Geometry: final body of the model. Coordinates: model frame, mm. Face numbers are marked on the shaded views. A direction names the side the tool comes from. Round coordinates to 2 decimals unless told otherwise and drop trailing zeros. Write each loop counter-clockwise with the first axis right and the second up, starting at its lowest first coordinate (ties: lowest second). Pieces come first, ordered by that corner, then holes. Notation, with made-up numbers: (-38, -7.5) -> (15, -7.5) arc R22 ccw to (15, 15.5) -> close; hole circle Ø8 at (72, 4.25). An arc over 180 degrees is marked (long way). One line per item, written item: value. Start each with the question number.
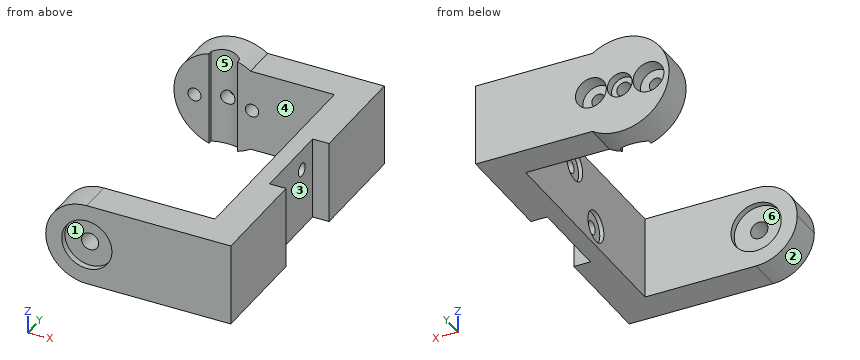
from build123d import *

# Parameters (mm, degrees)
SZKIC1_W                        = 45
SZKIC1_H                        = 20
SZKIC1_R                        = 2.1
DODANIE_WYCI_GNI_CIE1_DEPTH     = 8
SZKIC2_R                        = 6.1
WYTNIJ_WYCI_GNI_CIE1_DEPTH      = 1.5
WYTNIJ_WYCI_GNI_CIE2_START      = -1.5
SZKIC3_R                        = 6.1
WYTNIJ_WYCI_GNI_CIE2_DEPTH      = 1.5
SZKIC4_W                        = 8
SZKIC4_H                        = 20
DODANIE_WYCI_GNI_CIE2_DEPTH     = 56
ZAOKR_GLENIE1_R                 = 10
DODANIE_WYCI_GNI_CIE3_DEPTH     = 8
WYTNIJ_WYCI_GNI_CIE3_REACH      = 82.951
SZKIC6_R                        = 1.6
SZKIC7_R                        = 3.75
WYTNIJ_WYCI_GNI_CIE4_DEPTH      = 3.5
WYTNIJ_WYCI_GNI_CIE5_REACH      = 85.576
WYTNIJ_WYCI_GNI_CIE5_END_RADIUS = 12
SZKIC10_R                       = 3
WYTNIJ_WYCI_GNI_CIE6_DEPTH      = 2
WYTNIJ_WYCI_GNI_CIE7_REACH      = 81.177
WYTNIJ_WYCI_GNI_CIE7_END_RADIUS = 5
SZKIC11_R                       = 1.75
SZKIC12_W                       = 20
SZKIC12_H                       = 20.2
WYTNIJ_WYCI_GNI_CIE8_DEPTH      = 4
WYTNIJ_WYCI_GNI_CIE9_REACH      = 86.717
SZKIC13_R                       = 1.6
SZKIC14_R                       = 3.75
WYTNIJ_WYCI_GNI_CIE10_DEPTH     = 1


with BuildPart() as part:
    # Szkic1 → Dodanie-wyciągnięcie1 (new body)
    with BuildSketch(Plane(origin=(0, 0, 0), x_dir=(1, 0, 0), z_dir=(0, 1, 0))):
        with Locations((12.5, 0)):
            Rectangle(SZKIC1_W, SZKIC1_H)
        with Locations(Location((0, 0, 0), (0, 0, 270))):
            Circle(SZKIC1_R, mode=Mode.SUBTRACT)
    extrude(amount=DODANIE_WYCI_GNI_CIE1_DEPTH)

    # Szkic2 → Wytnij-wyciągnięcie1 (cut)
    with BuildSketch(Plane(origin=(0, 8, 0), x_dir=(1, 0, 0), z_dir=(0, 1, 0))):
        with Locations(Location((0, 0, 0), (0, 0, 270))):
            Circle(SZKIC2_R)
    extrude(amount=-WYTNIJ_WYCI_GNI_CIE1_DEPTH, mode=Mode.SUBTRACT)

    # Szkic3 → Wytnij-wyciągnięcie2 (cut)
    with BuildSketch(Plane.XZ.offset(WYTNIJ_WYCI_GNI_CIE2_START)):
        with Locations(Location((0, 0, 0), (0, 0, 90))):
            Circle(SZKIC3_R)
    extrude(amount=WYTNIJ_WYCI_GNI_CIE2_DEPTH, mode=Mode.SUBTRACT)

    # Szkic4 → Dodanie-wyciągnięcie2 (add)
    with BuildSketch(Plane(origin=(0, 8, 0), x_dir=(1, 0, 0), z_dir=(0, 1, 0))):
        with Locations((31, 0)):
            Rectangle(SZKIC4_W, SZKIC4_H)
    extrude(amount=DODANIE_WYCI_GNI_CIE2_DEPTH)

    # Zaokrąglenie1
    zaokr_glenie1_edges = [part.edges().sort_by_distance(p)[0] for p in [
        (-10, 4, -10),
        (-10, 4, 10),
    ]]
    fillet(zaokr_glenie1_edges, radius=ZAOKR_GLENIE1_R - 0.0001)  # a hair under: the kernel refuses the full size

    # Szkic5 → Dodanie-wyciągnięcie3 (add)
    with BuildSketch(Plane(origin=(0, 64, 0), x_dir=(1, 0, 0), z_dir=(0, 1, 0))):
        with BuildLine():
            Line((35, -10), (35, 10))
            Line((35, 10), (6.633249581, 10))
            ThreePointArc((6.633249581, 10), (-12, 0), (6.633249581, -10))
            Line((6.633249581, -10), (35, -10))
        make_face()
    extrude(amount=DODANIE_WYCI_GNI_CIE3_DEPTH)

    # Szkic6 → Wytnij-wyciągnięcie3 (cut, up to next)
    with BuildSketch(Plane(origin=(0, 72, 0), x_dir=(1, 0, 0), z_dir=(0, 1, 0)), mode=Mode.PRIVATE) as wytnij_wyci_gni_cie3_sk1:
        with Locations(Location((-7, 0, 0), (0, 0, 270))):
            Circle(SZKIC6_R)
    wytnij_wyci_gni_cie3_tool1 = extrude(wytnij_wyci_gni_cie3_sk1.sketch, amount=-WYTNIJ_WYCI_GNI_CIE3_REACH, mode=Mode.PRIVATE) & part.part
    # Szkic6 → Wytnij-wyciągnięcie3 (cut, up to next)
    with BuildSketch(Plane(origin=(0, 72, 0), x_dir=(1, 0, 0), z_dir=(0, 1, 0)), mode=Mode.PRIVATE) as wytnij_wyci_gni_cie3_sk2:
        with Locations(Location((7, 0, 0), (0, 0, 270))):
            Circle(SZKIC6_R)
    wytnij_wyci_gni_cie3_tool2 = extrude(wytnij_wyci_gni_cie3_sk2.sketch, amount=-WYTNIJ_WYCI_GNI_CIE3_REACH, mode=Mode.PRIVATE) & part.part
    add(wytnij_wyci_gni_cie3_tool1.solids().sort_by_distance((-7, 72, 0))[0], mode=Mode.SUBTRACT)
    add(wytnij_wyci_gni_cie3_tool2.solids().sort_by_distance((7, 72, 0))[0], mode=Mode.SUBTRACT)

    # Szkic7 → Wytnij-wyciągnięcie4 (cut)
    with BuildSketch(Plane(origin=(0, 72, 0), x_dir=(1, 0, 0), z_dir=(0, 1, 0))):
        with Locations(Location((7, 0, 0), (0, 0, 270))):
            Circle(SZKIC7_R)
        with Locations(Location((-7, 0, 0), (0, 0, 270))):
            Circle(SZKIC7_R)
    extrude(amount=-WYTNIJ_WYCI_GNI_CIE4_DEPTH, mode=Mode.SUBTRACT)

    # Wytnij-wyciągnięcie5: up to this cylinder (the profile starts inside it)
    wytnij_wyci_gni_cie5_end = Plane(origin=(0, 65.035303, 0), z_dir=(0, -1, 0)) * Cylinder(WYTNIJ_WYCI_GNI_CIE5_END_RADIUS, 196.152, mode=Mode.PRIVATE)
    # Szkic9 → Wytnij-wyciągnięcie5 (cut, up to the surface)
    with BuildSketch(Plane.XY.offset(12), mode=Mode.PRIVATE) as wytnij_wyci_gni_cie5_sk1:
        with BuildLine():
            Line((-3.5, 64), (3.5, 64))
            Line((3.5, 64), (3.5, 65))
            ThreePointArc((3.5, 65), (0, 66.429285786), (-3.5, 65))
            Line((-3.5, 65), (-3.5, 64))
        make_face()
    wytnij_wyci_gni_cie5_tool1 = extrude(wytnij_wyci_gni_cie5_sk1.sketch, amount=-WYTNIJ_WYCI_GNI_CIE5_REACH, mode=Mode.PRIVATE) & wytnij_wyci_gni_cie5_end
    add(wytnij_wyci_gni_cie5_tool1.solids().sort_by_distance((0, 65.035303, 12))[0], mode=Mode.SUBTRACT)

    # Szkic10 → Wytnij-wyciągnięcie6 (cut)
    with BuildSketch(Plane(origin=(0, 72, 0), x_dir=(1, 0, 0), z_dir=(0, 1, 0))):
        with Locations(Location((0, 0, 0), (0, 0, 270))):
            Circle(SZKIC10_R)
    extrude(amount=-WYTNIJ_WYCI_GNI_CIE6_DEPTH, mode=Mode.SUBTRACT)

    # Wytnij-wyciągnięcie7: up to this cylinder (the profile starts outside it)
    wytnij_wyci_gni_cie7_end = Plane(origin=(0, 61.429285786, 0), z_dir=(0, 0, 1)) * Cylinder(WYTNIJ_WYCI_GNI_CIE7_END_RADIUS, 173.354, mode=Mode.PRIVATE)
    # Szkic11 → Wytnij-wyciągnięcie7 (cut, up to the surface)
    with BuildSketch(Plane(origin=(0, 70, 0), x_dir=(1, 0, 0), z_dir=(0, 1, 0)), mode=Mode.PRIVATE) as wytnij_wyci_gni_cie7_sk1:
        with Locations(Location((0, 0, 0), (0, 0, 270))):
            Circle(SZKIC11_R)
    wytnij_wyci_gni_cie7_tool1 = extrude(wytnij_wyci_gni_cie7_sk1.sketch, amount=-WYTNIJ_WYCI_GNI_CIE7_REACH, mode=Mode.PRIVATE) - wytnij_wyci_gni_cie7_end
    add(wytnij_wyci_gni_cie7_tool1.solids().sort_by_distance((0, 70, 0))[0], mode=Mode.SUBTRACT)

    # Szkic12 → Wytnij-wyciągnięcie8 (cut)
    with BuildSketch(Plane(origin=(35, 0, 0), x_dir=(0, 0, -1), z_dir=(1, 0, 0))):
        with Locations((0, 36)):
            Rectangle(SZKIC12_W, SZKIC12_H)
    extrude(amount=-WYTNIJ_WYCI_GNI_CIE8_DEPTH, mode=Mode.SUBTRACT)

    # Szkic13 → Wytnij-wyciągnięcie9 (cut, up to next)
    with BuildSketch(Plane(origin=(31, 0, 0), x_dir=(0, 0, -1), z_dir=(1, 0, 0)), mode=Mode.PRIVATE) as wytnij_wyci_gni_cie9_sk1:
        with Locations((-5, 41)):
            Circle(SZKIC13_R)
    wytnij_wyci_gni_cie9_tool1 = extrude(wytnij_wyci_gni_cie9_sk1.sketch, amount=-WYTNIJ_WYCI_GNI_CIE9_REACH, mode=Mode.PRIVATE) & part.part
    # Szkic13 → Wytnij-wyciągnięcie9 (cut, up to next)
    with BuildSketch(Plane(origin=(31, 0, 0), x_dir=(0, 0, -1), z_dir=(1, 0, 0)), mode=Mode.PRIVATE) as wytnij_wyci_gni_cie9_sk2:
        with Locations((5.0495025, 31.049997525)):
            Circle(SZKIC13_R)
    wytnij_wyci_gni_cie9_tool2 = extrude(wytnij_wyci_gni_cie9_sk2.sketch, amount=-WYTNIJ_WYCI_GNI_CIE9_REACH, mode=Mode.PRIVATE) & part.part
    add(wytnij_wyci_gni_cie9_tool1.solids().sort_by_distance((31, 41, 5))[0], mode=Mode.SUBTRACT)
    add(wytnij_wyci_gni_cie9_tool2.solids().sort_by_distance((31, 31.049998, -5.049502))[0], mode=Mode.SUBTRACT)

    # Szkic14 → Wytnij-wyciągnięcie10 (cut)
    with BuildSketch(Plane.ZY.offset(-27)):
        with Locations((5, 41)):
            Circle(SZKIC14_R)
        with Locations((-5.0495025, 31.049997525)):
            Circle(SZKIC14_R)
    extrude(amount=-WYTNIJ_WYCI_GNI_CIE10_DEPTH, mode=Mode.SUBTRACT)


solid = part.part
(1) Pin query (flat end, axial travel): pin 1 (4 mm diameter, centred on y = 34.5, z = -2.5, fed in from +X); pin 2 (8 mm diameter, centred on x = 0, z = 0, fed in from -Y); pin 3 (4.5 mm diameter, centred on y = 41, z = 5, fed in from -X). Return the tip coordinate at first contact, or that it passes through.
(2) Set-up query: the marked faces 4, 5 and 6. Return all of +Z, -Z, +X, -X, +Y, -Y with unobstructed straight access to the full face (end or side cutting, diameter ignored); none if empty.
(3) Section query B-B (y = 41). Output: boundary loops of the cut face in (x, z), and give its area (3 significant figures).
(4) Line query: probe 1 along X at (y, z) = (71.2, 0); probe 2 along X at (y, z) = (69.15, 0); probe 3 along Y at (x, z) = (4.5, -4.5). Output: solid intervals per line, ascending.
(5) Pull-direction query (Z, two-part tool) for the marked faces 1, 2 and 3; classes: pulls with the +Z half, pulls with the -Z half, needs draft (parallel to the pull), parting line crosses it, or undercut.
(6) Section query A-A (x = 32). Output: boundary loops of the cut face in (y, z), and give its area (3 significant figures).
(7) Section query D-D (x = -7). Output: boundary loops of the cut face in (y, z), and give its area (3 significant figures).
Results list:
1. pin 1: stops at x = 31
1. pin 2: stops at y = 1.5
1. pin 3: stops at x = 28
2. face 4: +Z, -Z, -X
2. face 5: +Z, -Z
2. face 6: none
3. outline: (27, -10) -> (31, -10) -> (31, 3.4) -> (28, 3.4) -> (28, 1.25) -> (27, 1.25) -> close; (27, 8.75) -> (28, 8.75) -> (28, 6.6) -> (31, 6.6) -> (31, 10) -> (27, 10) -> close
3. area: 62.9 mm^2
4. probe 1: x = -12 to -10.75, -3.25 to -3, 3 to 3.25, 10.75 to 35
4. probe 2: x = -12 to -10.75, -3.25 to -1.75, 1.75 to 3.25, 10.75 to 35
4. probe 3: y = 0 to 8, 64 to 72
5. face 1: undercut
5. face 2: pulls with the -Z half
5. face 3: needs draft
6. outline: (0, -10) -> (25.9, -10) -> (25.9, 10) -> (0, 10) -> close; (46.1, -10) -> (72, -10) -> (72, 10) -> (46.1, 10) -> close
6. area: 1,040 mm^2
7. outline: (0, -7.14) -> (8, -7.14) -> (8, 7.14) -> (0, 7.14) -> close; (64, -9.75) -> (72, -9.75) -> (72, -3.75) -> (68.5, -3.75) -> (68.5, -1.6) -> (64, -1.6) -> close; (64, 1.6) -> (68.5, 1.6) -> (68.5, 3.75) -> (72, 3.75) -> (72, 9.75) -> (64, 9.75) -> close
7. area: 230 mm^2
